```python
from build123d import *

# Parameters (mm, degrees)
SKETCH1_W           = 300
SKETCH1_H           = 52
BOSS_EXTRUDE2_DEPTH = 3
SKETCH2_W           = 20
SKETCH2_H           = 3
CUT_EXTRUDE1_DEPTH  = 10
SKETCH3_W           = 20
SKETCH3_H           = 3
CUT_EXTRUDE4_DEPTH  = 10
SKETCH4_W           = 20
SKETCH4_H           = 3
CUT_EXTRUDE5_DEPTH  = 10


with BuildPart() as part:
    # Sketch1 → Boss-Extrude2 (new body)
    with BuildSketch(Plane.XY):
        Rectangle(SKETCH1_W, SKETCH1_H)
    extrude(amount=BOSS_EXTRUDE2_DEPTH)

    # Sketch2 → Cut-Extrude1 (cut)
    with BuildSketch(Plane.XY.offset(3)):
        with Locations((-100, 24.5)):
            Rectangle(SKETCH2_W, SKETCH2_H)
    extrude(amount=-CUT_EXTRUDE1_DEPTH, mode=Mode.SUBTRACT)

    # Sketch3 → Cut-Extrude4 (cut)
    with BuildSketch(Plane.XY.offset(3)):
        with Locations((-100, -24.5)):
            Rectangle(SKETCH3_W, SKETCH3_H)
        with Locations((100, -24.5)):
            Rectangle(SKETCH3_W, SKETCH3_H)
    extrude(amount=-CUT_EXTRUDE4_DEPTH, mode=Mode.SUBTRACT)

    # Sketch4 → Cut-Extrude5 (cut)
    with BuildSketch(Plane.XY.offset(3)):
        with Locations((50, 24.5)):
            Rectangle(SKETCH4_W, SKETCH4_H)
    extrude(amount=-CUT_EXTRUDE5_DEPTH, mode=Mode.SUBTRACT)


solid = part.part
```
Model file for the job. Use its own axes, mm. Coordinates: 2 decimals unless noted, no trailing zeros. Order: outer loops, then holes, each group sorted by start corner. A loop starts at its lowest first (then second) coordinate and runs counter-clockwise, first axis right, second up. Notation, with made-up numbers: M 6.5,84.5 L 22.5,84.5 A31 cw 22.5,119.5 Z; hole C 60,-16 d7. An arc over 180 degrees is marked long. Answer as CSV lines item,"result".
(1) Band-saw the part on A-A, the plane z = 0.5. List the corners of the cut face in (x, y).
Geometry says:
outline,"M -150,-26 L -110,-26 L -110,-23 L -90,-23 L -90,-26 L 90,-26 L 90,-23 L 110,-23 L 110,-26 L 150,-26 L 150,26 L 60,26 L 60,23 L 40,23 L 40,26 L -90,26 L -90,23 L -110,23 L -110,26 L -150,26 Z"
(2) Band-saw the part on B-B, the plane x = 104.5. List the corners of the cut face in (y, z).
Geometry says:
outline,"M -23,0 L 26,0 L 26,3 L -23,3 Z"
(3) Wall check: line 1 along Y through (x, z) = (51.5, 1.65); line 2 along Y through (x, z) = (92, 1.4). Give the ranges that are in metal, low to high.
Geometry says:
line 1,"y = -26 to 23"
line 2,"y = -23 to 26"
(4) Flat gauge pins, fed straight in: pin 1 (0.9 mm diameter, centred on x = -103, z = 1.5, fed in from +Y); pin 2 (1.5 mm diameter, centred on x = -98.5, z = 1, fed in from -Y). Where does each tip first touch, or does it go through?
Geometry says:
pin 1,"stops at y = 23"
pin 2,"stops at y = -23"
